Can you work these out from the model? Positions are in its coordinate system, mm. Face numbers are marked on the shaded views. A direction names the side the tool comes from. Round coordinates to 2 decimals unless told otherwise and drop trailing zeros. Write each loop counter-clockwise with the first axis right and the second up, starting at its lowest first coordinate (ties: lowest second). Pieces come first, ordered by that corner, then holes. Notation, with made-up numbers: M 36.25,83.25 L 66.25,83.25 A31 cw 66.25,110.25 Z; hole C 73.5,85 d1. An arc over 180 degrees is marked long. Answer as a JSON object with one key per item and string values. Group by question number.
1) Suppose I cut it at A-A, the plane x = -4.05. Write out the boundary of the cut face in (y, z), and give its area (3 significant figures).
2) Suppose I cut it at D-D, the plane y = -5. Write out the boundary of the cut face in (x, z).
3) Please list where these lines run through material, in increasing order: L1, parallel to Y at x = 13, z = -11; L2, parallel to Y at x = -4.05, z = 0.6; L3, parallel to X at y = -8.5, z = -2.5. Write a range as [from, to].
4) I'm going to push flat-ended pins straight in: pin 1 Ø1 at (y, z) = (1, -3) entering from -X; pin 2 Ø1.4 at (x, z) = (-20.5, -2.5) entering from +Y (3 decimals); pin 3 Ø1.2 at (x, z) = (-13, 1) entering from +Y; pin 4 Ø1 at (y, z) = (-2.5, -9) entering from +X. Where does each tip first touch, or does it pass through?
5) Suppose I cut it at C-C, the plane z = -5.5. Write out the boundary of the cut face in (x, y) (3 decimals), and give its area (3 significant figures).
6) On a 3-axis mill with a long thin cutter (end or side, diameter ignored), from which of +Z, -Z, +X, -X, +Y, -Y can I reach the whole of each face in a straight line? I mean the marked faces 4, 5, 6 and 7. Say none if no direction works.
7) If we mould it in two halves opening along Y, with no side actions, what happens to the marked faces 1, 2 and 3? For each: +Y half, -Y half, draft (parallel to the pull), parting line (faces both ways), or undercut.
8) Suppose I cut it at B-B, the plane y = 0. Write out the boundary of the cut face in (x, z).
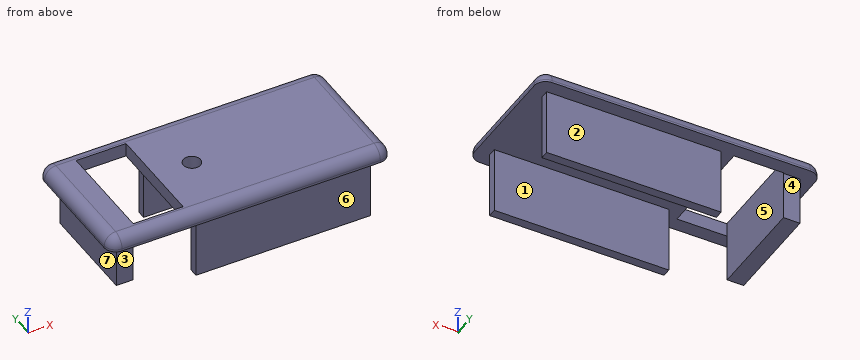
Autodesk Inventor part; units mm, degrees
ref_plane "Work Plane4" through (-22.25, -9, -8.6) normal (0, 0, 1) x (1, 0, 0)
ref_plane "YZ Plane" through (0, 0, 0) normal (1, 0, 0) x (0, 1, 0)
ref_plane "XZ Plane" through (0, 0, 0) normal (0, 1, 0) x (-1, 0, 0)
ref_plane "Work Plane1" through (0, 0, 0) normal (0, 0, 1) x (1, 0, 0)
sketch "Sketch1" plane through (0, 0, 0) normal (0, 0, 1) x (1, 0, 0)
  arc A0 (-22.65, 11.4) -> (-24.65, 9.4) centre (-22.65, 9.4) ccw
  line L0 (-24.65, 9.4) -> (-24.65, -9.4)
  arc A1 (-24.65, -9.4) -> (-22.65, -11.4) centre (-22.65, -9.4) ccw
  line L1 (-22.65, -11.4) -> (22.65, -11.4)
  arc A2 (22.65, -11.4) -> (24.65, -9.4) centre (22.65, -9.4) ccw
  line L2 (24.65, -9.4) -> (24.65, 9.4)
  arc A3 (24.65, 9.4) -> (22.65, 11.4) centre (22.65, 9.4) ccw
  line L3 (22.65, 11.4) -> (-22.65, 11.4)
  line L4 (22.25, 9) -> (22.25, -9)
  line L5 (22.25, -9) -> (-8.35, -9)
  line L6 (-8.35, -2.5) -> (-8.35, -9)
  line L7 (-10.6, -2.5) -> (-8.35, -2.5)
  line L8 (-10.6, -9) -> (-10.6, -2.5)
  line L9 (-10.6, -9) -> (-22.25, -9)
  line L10 (-22.25, -9) -> (-22.25, 9)
  line L11 (-22.25, 9) -> (-10.6, 9)
  line L12 (-10.6, 2.5) -> (-10.6, 9)
  line L13 (-8.35, 2.5) -> (-10.6, 2.5)
  line L14 (-8.35, 9) -> (-8.35, 2.5)
  line L15 (-8.35, 9) -> (22.25, 9)
  line L16 (-20.5, -9) -> (-20.5, -4.5)
  line L17 (-20.5, 4.5) -> (-20.5, 9)
  line L18 (-20.5, -4.5) -> (-20.5, 4.5)
  line L19 (-10.6, -2.5) -> (-10.6, 2.5)
  line L20 (22.25, -7.5) -> (-8.35, -7.5)
  line L21 (-8.35, 7.5) -> (22.25, 7.5)
  point P0 (0, 0)
  dimension "d0" = 1.5
  dimension "d1" = 1.5
ref_plane "Work Plane2" through (0, 0, -11.8) normal (0, 0, 1) x (1, 0, 0)
extrude "Extrusion1" add sketch "Sketch1" against normal up to surface (11.8 mm away) contours L4 L21 L14 L15 | L4 L5 L6 L20
ref_plane "Work Plane3" through (0, 0, 0) normal (0, 0, 1) x (1, 0, 0)
sketch "Sketch2" plane through (0, 0, 0) normal (0, 0, 1) x (1, 0, 0)
  line L0 (-22.25, -9) -> (-22.25, 9)
  line L1 (-10.6, -9) -> (-10.6, -2.5)
  line L2 (-10.6, 2.5) -> (-10.6, 9)
  line L3 (-10.6, -2.5) -> (-10.6, 2.5)
  line L4 (-10.6, -8.875) -> (-19.35, -8.875)
  line L5 (-19.35, -8.875) -> (-19.35, 8.875)
  line L6 (-19.35, 8.875) -> (-10.6, 8.875)
  line L7 (-10.6, 8.875) -> (-10.6, -8.875)
  line L8 (-19.35, -8.875) -> (-22.25, -8.875)
  line L9 (-19.35, 8.875) -> (-22.25, 8.875)
  point P0 (0, 0)
  point P1 (-10.6, 0)
  dimension "d4" = 17.75
  dimension "d5" = 8.75
ref_plane "Work Plane4" through (-22.25, -9, -8.6) normal (0, 0, 1) x (1, 0, 0)
extrude "Extrusion2" add sketch "Sketch2" against normal up to surface (8.6 mm away) contours L0 L9 L5 L8
sketch "Sketch3" plane through (0, 0, 0) normal (0, 0, 1) x (1, 0, 0)
  arc A0 (-22.65, 11.4) -> (-24.65, 9.4) centre (-22.65, 9.4) ccw
  line L0 (-24.65, 9.4) -> (-24.65, -9.4)
  arc A1 (-24.65, -9.4) -> (-22.65, -11.4) centre (-22.65, -9.4) ccw
  line L1 (-22.65, -11.4) -> (22.65, -11.4)
  arc A2 (22.65, -11.4) -> (24.65, -9.4) centre (22.65, -9.4) ccw
  line L2 (24.65, -9.4) -> (24.65, 9.4)
  arc A3 (24.65, 9.4) -> (22.65, 11.4) centre (22.65, 9.4) ccw
  line L3 (22.65, 11.4) -> (-22.65, 11.4)
  line L4 (22.25, 9) -> (22.25, -9)
  line L5 (22.25, -9) -> (-8.35, -9)
  line L6 (-8.35, -2.5) -> (-8.35, -9)
  line L7 (-10.6, -2.5) -> (-8.35, -2.5)
  line L8 (-10.6, -9) -> (-10.6, -2.5)
  line L9 (-10.6, -9) -> (-22.25, -9)
  line L10 (-22.25, -9) -> (-22.25, 9)
  line L11 (-22.25, 9) -> (-10.6, 9)
  line L12 (-10.6, 2.5) -> (-10.6, 9)
  line L13 (-8.35, 2.5) -> (-10.6, 2.5)
  line L14 (-8.35, 9) -> (-8.35, 2.5)
  line L15 (-8.35, 9) -> (22.25, 9)
  line L16 (-19.35, -8.875) -> (-19.35, 8.875)
  line L17 (-19.35, -9) -> (-10.6, -9)
  line L18 (-10.6, -9) -> (-10.6, 9)
  line L19 (-10.6, 9) -> (-19.35, 9)
  line L20 (-19.35, 9) -> (-19.35, -9)
  point P0 (0, 0)
  point P1 (-19.35, 0)
extrude "Extrusion3" add sketch "Sketch3" along normal blind 2.4 contours L3 A3 L2 A2 L1 A1 L0 A0 | L4 L5 L6 L7 L18 L13 L14 L15 | L20 L16 L9 L10 L11
fillet "Fillet1" radius 2 8 edges at (-24.0642, 10.8142, 2.4) (-24.65, 0, 2.4) (-24.0642, -10.8142, 2.4) (0, -11.4, 2.4) (24.0642, -10.8142, 2.4) (24.65, 0, 2.4) (24.0642, 10.8142, 2.4) (0, 11.4, 2.4)
sketch "Sketch4" plane through (0, 0, 2.4) normal (0, 0, 1) x (1, 0, 0)
  line L0 (22.25, 9) -> (22.25, -9)
  line L1 (22.25, -9) -> (-8.35, -9)
  line L2 (-8.35, -2.5) -> (-8.35, -9)
  circle A0 centre (-4.05, 0) radius 1.5
  line L3 (22.25, 0) -> (28.5402, 0) construction
  point P0 (0, 0)
  dimension "d11" = 3
  dimension "d12" = 4.3
extrude "Extrusion4" cut sketch "Sketch4" against normal up to surface (2.4 mm away)
equation "\"d1\" = d0"
properties part number "rf_tester_top"
Results:
{
 "1": {"outline": "M -11.4,0 L -9,0 L -9,-11.8 L -7.5,-11.8 L -7.5,0 L -1.5,0 L -1.5,2.4 L -9.4,2.4 A2 ccw -11.4,0.4 Z; M 1.5,0 L 7.5,0 L 7.5,-11.8 L 9,-11.8 L 9,0 L 11.4,0 L 11.4,0.4 A2 ccw 9.4,2.4 L 1.5,2.4 Z", "area": "81.2 mm^2"},
 "2": {"outline": "M -24.65,0 L -22.25,0 L -22.25,-8.6 L -19.35,-8.6 L -19.35,2.4 L -22.65,2.4 A2 ccw -24.65,0.4 Z; M -10.6,0 L 24.65,0 L 24.65,0.4 A2 ccw 22.65,2.4 L -10.6,2.4 Z"},
 "3": {"L1": "[-9, -7.5], [7.5, 9]", "L2": "[-11.39, -1.5], [1.5, 11.39]", "L3": "[-22.25, -19.35], [-8.35, 22.25]"},
 "4": {"pin 1": "x = -22.25", "pin 2": "y = 8.875", "pin 3": "y = 11.4", "pin 4": "x = -19.35"},
 "5": {"outline": "M -22.25,-8.875 L -19.35,-8.875 L -19.35,8.875 L -22.25,8.875 Z; M -8.35,-9 L 22.25,-9 L 22.25,-7.5 L -8.35,-7.5 Z; M -8.35,7.5 L 22.25,7.5 L 22.25,9 L -8.35,9 Z", "area": "143 mm^2"},
 "6": {"face 4": "-Z, -X, +Y", "face 5": "+Z, -Z", "face 6": "-Z, +X, -X, -Y", "face 7": "-Z, -X, +Y, -Y"},
 "7": {"face 1": "undercut", "face 2": "+Y half", "face 3": "-Y half"},
 "8": {"outline": "M -24.65,0 L -22.25,0 L -22.25,-8.6 L -19.35,-8.6 L -19.35,2.4 L -22.65,2.4 A2 ccw -24.65,0.4 Z; M -10.6,0 L -5.55,0 L -5.55,2.4 L -10.6,2.4 Z; M -2.55,0 L 24.65,0 L 24.65,0.4 A2 ccw 22.65,2.4 L -2.55,2.4 Z"}
}
